For this review, take the finished solid that the model builds, in its own axes (mm). Face numbers are marked on the shaded views. Coordinates: 2 decimals unless noted, no trailing zeros. Write each loop counter-clockwise with the first axis right and the second up, starting at its lowest first coordinate (ties: lowest second). Pieces come first, ordered by that corner, then holes. Notation, with made-up numbers: M 84.25,-11.5 L 114.25,-11.5 A16 cw 114.25,19.5 Z; hole C 46.25,-2.75 d7. An arc over 180 degrees is marked long. One line per question, with ' | ' between items.
from build123d import *


with BuildPart() as part:
    # Esquisse1 → Base-Révolution (revolve)
    with BuildSketch(Plane.XY, mode=Mode.PRIVATE) as base_r_volution_sk:
        with BuildLine():
            Line((3.5, 4.5), (3.5, 5.8))
            Line((3.5, 5.8), (1.053565375, 5.8))
            ThreePointArc((1.053565375, 5.8), (0, 5.5), (-1.053565375, 5.8))
            Line((-1.053565375, 5.8), (-3.5, 5.8))
            Line((-3.5, 5.8), (-3.5, 4.5))
            ThreePointArc((-3.5, 4.5), (-3.353553391, 4.146446609), (-3, 4))
            Line((-3, 4), (3, 4))
            ThreePointArc((3, 4), (3.353553391, 4.146446609), (3.5, 4.5))
        make_face()
    revolve(base_r_volution_sk.sketch.rotate(Axis((-4.370908092, 0, 0), (1, 0, 0)), 90), axis=Axis((-4.370908092, 0, 0), (1, 0, 0)))


solid = part.part
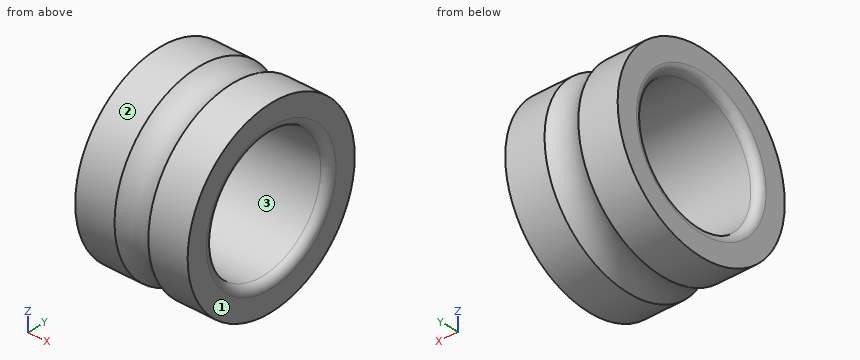
1) The part is to be moulded in two halves that separate along Z. For the marked faces 1, 2 and 3, say which applies: +Z half, -Z half, draft (parallel to the pull), parting line (faces both ways), or undercut.
Responses:
face 1: draft | face 2: parting line | face 3: undercut
2) To check wall thickness, follow line 1 along Y through (x, z) = (2.25, 0); line 2 along Y through (x, z) = (-0.9, 0); line 3 along X through (y, z) = (4.5, 3.5). State the ranges of each line that lie inside material, in increasing order. Write a range as [from, to].
Responses:
line 1: [-5.8, -4], [4, 5.8] | line 2: [-5.71, -4], [4, 5.71] | line 3: [-3.5, -0.87], [0.87, 3.5]
3) Insertion check: pin 1 Ø1 at (x, y) = (2.5, -2) entering from -Z; pin 2 Ø1 at (x, y) = (0, 2) entering from -Z; pin 3 Ø4 at (x, z) = (-1, -4) entering from -Y; pin 4 Ø2 at (y, z) = (2.5, -1) entering from +X. Each pin has a flat end and moves straight along its axis. Give the tip position at first contact, or say it passes through.
Responses:
pin 1: z = -5.6 | pin 2: z = -5.29 | pin 3: y = -5.44 | pin 4: through
4) We need section A-A on y = 0. State the section outline as (x, z) points.
Responses:
outline: M -3.5,-5.8 L -1.05,-5.8 A2 cw 1.05,-5.8 L 3.5,-5.8 L 3.5,-4.5 A0.5 ccw 3,-4 L -3,-4 A0.5 ccw -3.5,-4.5 Z; M -3.5,4.5 A0.5 ccw -3,4 L 3,4 A0.5 ccw 3.5,4.5 L 3.5,5.8 L 1.05,5.8 A2 cw -1.05,5.8 L -3.5,5.8 Z
5) We need section C-C on x = -1.75. State the section outline as (y, z) points, then the cut area to 3 significant figures.
Responses:
outline: C 0,0 d11.6; hole C 0,0 d8 | area: 55.4 mm^2
